Could you check a few things on this model? Use its own coordinates, in mm. A direction names the side the tool comes from. Coordinates: 2 decimals unless noted, no trailing zeros. Loops run counter-clockwise (first coordinate to the right, second up) from the corner with the lowest first, then second, coordinate; pieces in that order, holes last. Notation, with made-up numbers: (39.25, 51.5) - (71.25, 51.5) arc R36 cw to (71.25, 85.5) - close; hole circle Ø1 at (55, 64.5). An arc over 180 degrees is marked (long way). Use CSV: the item, a comma, the result in double quotes.
Autodesk Inventor part; units mm, degrees
ref_plane "YZ Plane" through (0, 0, 0) normal (1, 0, 0) x (0, 1, 0)
ref_plane "XZ Plane" through (0, 0, 0) normal (0, 1, 0) x (-1, 0, 0)
ref_plane "XY Plane" through (0, 0, 0) normal (0, 0, 1) x (1, 0, 0)
sketch "Sketch1" plane through (0, 0, 0) normal (0, 0, 1) x (1, 0, 0)
  line L0 (-2.5, -7) -> (-2.5, -47)
  line L1 (-3.5, 0) -> (-3.5, -7)
  line L2 (-3.5, -7) -> (-2.5, -7)
  line L3 (-2, -47) -> (-2, -57)
  line L4 (-2.5, -47) -> (-2, -47)
  line L5 (-2, -57) -> (0, -57)
  line L6 (-3.5, 0) -> (0, 0)
  line L7 (0, 0) -> (0, -59)
  dimension "d1" = 7
  dimension "d3" = 40
  dimension "d5" = 10
revolve "Revolution1" add sketch "Sketch1" angle 360 about axis through (0, 0, 0) along (0, -1, 0)
thread "Thread1"
sketch "Sketch2" plane through (0, 0, 0) normal (1, 0, 0) x (0, 1, 0)
  line L0 (-7, 3.5) -> (-7, -3.5)
  line L1 (0, 3.5) -> (0, -3.5)
  circle A0 centre (-3.5, 0) radius 1.5
  point P0 (0, 0)
  dimension "d11" = 3
  dimension "d12" = 3.5
  dimension "d13" = 3.5
extrude "Extrusion1" add sketch "Sketch2" along normal mid plane 23
properties part number "HUDSON-1-84"
(1) Suppose I cut it at B-B (z = 0). Write out the boundary of the cut face in (x, y).
Computed:
outline,"(-11.5, -5) - (-3.5, -5) - (-3.5, -7) - (-2.5, -7) - (-2.5, -47) - (-2, -47) - (-2, -57) - (2, -57) - (2, -47) - (2.5, -47) - (2.5, -7) - (3.5, -7) - (3.5, -5) - (11.5, -5) - (11.5, -2) - (3.5, -2) - (3.5, 0) - (-3.5, 0) - (-3.5, -2) - (-11.5, -2) - close"
(2) Please list where these lines run through material, in increasing order: line 1 (X direction, y = -7.5, z = -1.5); line 2 (X direction, y = -20, z = -0.25).
Computed:
line 1,"x = -2 to 2"
line 2,"x = -2.49 to 2.49"
(3) Suppose I cut it at D-D (y = -12). Write out the boundary of the cut face in (x, z).
Computed:
outline,"circle Ø5 at (0, 0)"
(4) Which directions (+Z, -Z, +X, -X, +Y, -Y) give clear straight access to the entire face, cutting with the end or side of a thin tool? Please do faces 1 (the face through (2.8, -3.5, 2.1)), 2 (the face through (0, -52, 2)), 3 (the face through (0, 0, 0)), 4 (the face through (7.273, -2.114, 0.575)), 5 (the face through (-7.273, -2.114, -0.575)).
Computed:
face 1,"none"
face 2,"-Y"
face 3,"+Z, -Z, +X, -X, +Y"
face 4,"+X"
face 5,"-X"
(5) Suppose I cut it at A-A (y = -3.5). Write out the boundary of the cut face in (x, z), plus the area to 3 significant figures.
Computed:
outline,"(-11.5, -1.5) - (-3.16, -1.5) arc R3.5 ccw to (3.16, -1.5) - (11.5, -1.5) - (11.5, 1.5) - (3.16, 1.5) arc R3.5 ccw to (-3.16, 1.5) - (-11.5, 1.5) - close"
area,"87.1 mm²"
(6) Suppose I cut it at C-C (x = 0). Write out the boundary of the cut face in (y, z).
Computed:
outline,"(-57, -2) - (-47, -2) - (-47, -2.5) - (-7, -2.5) - (-7, -3.5) - (0, -3.5) - (0, 3.5) - (-7, 3.5) - (-7, 2.5) - (-47, 2.5) - (-47, 2) - (-57, 2) - close"
(7) Will these pins go through, and if not, where does the flat tip stop? pin 1 (8 mm diameter, centred on x = 0.5, y = -38, fed in from +Z); pin 2 (4 mm diameter, centred on x = 8, z = 1.5, fed in from +Y); pin 3 (5 mm diameter, centred on x = 1, y = -17.5, fed in from -Z).
Computed:
pin 1,"stops at z = 2.5"
pin 2,"stops at y = -2"
pin 3,"stops at z = -2.5"
